from build123d import *

# Parameters (mm, degrees)
SKETCH1_W                 = 146.05
SKETCH1_H                 = 266.7
BOSS_EXTRUDE1_DEPTH       = 15.875
SKETCH2_W                 = 110.49
SKETCH2_H                 = 224.79
CUT_EXTRUDE1_DEPTH        = 2.54
CUT_EXTRUDE2_DEPTH        = 10.16
F_4_40_TAPPED_HOLE1_D     = 2.2606
F_4_40_TAPPED_HOLE1_DEPTH = 10.16
F_4_40_TAPPED_HOLE1_TIP   = 0.679152758
F_8_CLEARANCE_HOLE1_D     = 4.9149
F_8_32_TAPPED_HOLE1_D     = 3.4544
F_8_32_TAPPED_HOLE1_DEPTH = 12.7
F_8_32_TAPPED_HOLE1_TIP   = 1.037806461
F_4_40_TAPPED_HOLE2_D     = 2.2606
F_4_40_TAPPED_HOLE2_DEPTH = 10.16
F_4_40_TAPPED_HOLE2_TIP   = 0.679152758


with BuildPart() as part:
    # Sketch1 → Boss-Extrude1 (new body)
    with BuildSketch(Plane(origin=(0, 0, 0), x_dir=(1, 0, 0), z_dir=(0, 1, 0))):
        with Locations((73.025, 133.35)):
            Rectangle(SKETCH1_W, SKETCH1_H)
    extrude(amount=BOSS_EXTRUDE1_DEPTH)

    # Sketch2 → Cut-Extrude1 (cut)
    with BuildSketch(Plane(origin=(0, 15.875, 0), x_dir=(1, 0, 0), z_dir=(0, 1, 0))):
        with Locations((60.96, 130.81)):
            Rectangle(SKETCH2_W, SKETCH2_H)
    extrude(amount=-CUT_EXTRUDE1_DEPTH, mode=Mode.SUBTRACT)

    # Sketch3 → Cut-Extrude2 (cut)
    with BuildSketch(Plane(origin=(0, 13.335, 0), x_dir=(1, 0, 0), z_dir=(0, 1, 0))):
        Polygon((19.685, 26.035), (19.685, 18.415), (5.715, 18.415), (5.715, 32.385), (13.335, 32.385), (13.335, 121.285), (19.685, 121.285), (19.685, 133.985), (5.715, 133.985), (5.715, 243.205), (19.685, 243.205), (19.685, 235.585), (37.8587, 235.585), (37.8587, 26.035), align=None)
        Polygon((44.2087, 26.035), (102.235, 26.035), (102.235, 18.415), (116.205, 18.415), (116.205, 32.385), (108.585, 32.385), (108.585, 121.285), (102.235, 121.285), (102.235, 133.985), (108.585, 133.985), (108.585, 229.235), (116.205, 229.235), (116.205, 243.205), (102.235, 243.205), (102.235, 235.585), (44.2087, 235.585), align=None)
    extrude(amount=-CUT_EXTRUDE2_DEPTH, mode=Mode.SUBTRACT)

    # #4-40 Tapped Hole1
    with Locations(Plane(origin=(0, 13.335, 0), x_dir=(1, 0, 0), z_dir=(0, 1, 0))):
        with Locations((108.585, 127.635), (13.335, 127.635)):
            Hole(F_4_40_TAPPED_HOLE1_D / 2, depth=F_4_40_TAPPED_HOLE1_DEPTH)
            with Locations((0, 0, -(F_4_40_TAPPED_HOLE1_DEPTH + F_4_40_TAPPED_HOLE1_TIP / 2))):  # 118° drill point
                Cone(0, F_4_40_TAPPED_HOLE1_D / 2, F_4_40_TAPPED_HOLE1_TIP, mode=Mode.SUBTRACT)

    # #8 Clearance Hole1 (through all)
    with Locations(Plane(origin=(0, 15.875, 0), x_dir=(1, 0, 0), z_dir=(0, 1, 0))):
        with Locations((12.7, 6.35), (139.7, 6.35), (139.7, 260.35), (12.7, 260.35)):
            Hole(F_8_CLEARANCE_HOLE1_D / 2)

    # #8-32 Tapped Hole1
    with Locations(Plane(origin=(0, 15.875, 0), x_dir=(1, 0, 0), z_dir=(0, 1, 0))):
        with Locations((44.2087, 6.35), (44.2087, 260.35), (139.7, 133.35)):
            Hole(F_8_32_TAPPED_HOLE1_D / 2, depth=F_8_32_TAPPED_HOLE1_DEPTH)
            with Locations((0, 0, -(F_8_32_TAPPED_HOLE1_DEPTH + F_8_32_TAPPED_HOLE1_TIP / 2))):  # 118° drill point
                Cone(0, F_8_32_TAPPED_HOLE1_D / 2, F_8_32_TAPPED_HOLE1_TIP, mode=Mode.SUBTRACT)

    # #4-40 Tapped Hole2
    with Locations(Plane(origin=(0, 15.875, 0), x_dir=(1, 0, 0), z_dir=(0, 1, 0))):
        with Locations((108.585, 249.555), (122.555, 26.035), (25.4, 249.555), (25.4, 12.065)):
            Hole(F_4_40_TAPPED_HOLE2_D / 2, depth=F_4_40_TAPPED_HOLE2_DEPTH)
            with Locations((0, 0, -(F_4_40_TAPPED_HOLE2_DEPTH + F_4_40_TAPPED_HOLE2_TIP / 2))):  # 118° drill point
                Cone(0, F_4_40_TAPPED_HOLE2_D / 2, F_4_40_TAPPED_HOLE2_TIP, mode=Mode.SUBTRACT)


solid = part.part
Geometry check sheet. Reference: the model listing, model coordinates, mm. A direction names the side the tool comes from. Give positions to 0.01 mm unless a question says otherwise; leave off trailing zeros. Order: outer loops, then holes, each group sorted by start corner. A loop starts at its lowest first (then second) coordinate and runs counter-clockwise, first axis right, second up. Notation, with made-up numbers: M 72,26 L 91,26 A34 ccw 91,61 Z; hole C 11.5,44 d11. An arc over 180 degrees is marked long. Use a Markdown table: item, result.
Item 1: Draft check along X on faces 3 (the flat face through (121, 15.875, -135)), 4 (the cylindrical face through (14.51, 7.83, -8.01)). Enter one of: +X half, -X half, draft (parallel to the pull), parting line (faces both ways), or undercut.
Answers follow:
| item | result |
|---|---|
| face 3 | draft |
| face 4 | undercut |
Item 2: Material ranges on line 1 along X through (y, z) = (7.75, -197.5) (3 decimals); line 2 along Z through (x, y) = (14.5, 14) (3 decimals); line 3 along Z through (x, y) = (11, 10.5) (3 decimals), recorded low to high.
Answers follow:
| item | result |
|---|---|
| line 1 | x = 0 to 5.715, 37.859 to 44.209, 108.585 to 146.05 |
| line 2 | z = -266.7 to -262.023, -258.677 to -243.205, -18.415 to -8.023, -4.677 to 0 |
| line 3 | z = -266.7 to -262.125, -258.575 to -243.205, -133.985 to -32.385, -18.415 to -8.125, -4.575 to 0 |
Item 3: Section check B-B (z = -222.5). Record the cut outline in (x, y) (3 decimals).
Answers follow:
| item | result |
|---|---|
| outline | M 0,0 L 146.05,0 L 146.05,15.875 L 116.205,15.875 L 116.205,13.335 L 108.585,13.335 L 108.585,3.175 L 44.209,3.175 L 44.209,13.335 L 37.859,13.335 L 37.859,3.175 L 5.715,3.175 L 5.715,15.875 L 0,15.875 Z |
Item 4: Depth check by flat-ended pin: P1, Ø6, axis at x = 43.5, z = -161.5, coming from the +Y side (3 decimals); P2, Ø2, axis at x = 34.5, z = -216.5, coming from the +Y side (3 decimals); P3, Ø4, axis at x = 12.7, z = -6.35, coming from the +Y side. Enter the tip coordinate at first touch or a pass-through.
Answers follow:
| item | result |
|---|---|
| P1 | stops at y = 13.335 |
| P2 | stops at y = 3.175 |
| P3 | passes through |
Item 5: Section check C-C (z = -58.5). Record the cut outline in (x, y) (3 decimals).
Answers follow:
| item | result |
|---|---|
| outline | M 0,0 L 146.05,0 L 146.05,15.875 L 116.205,15.875 L 116.205,13.335 L 108.585,13.335 L 108.585,3.175 L 44.209,3.175 L 44.209,13.335 L 37.859,13.335 L 37.859,3.175 L 13.335,3.175 L 13.335,13.335 L 5.715,13.335 L 5.715,15.875 L 0,15.875 Z |
Item 6: Tool access check on faces 1 (the flat face through (73, 8, -26.035)), 2 (the flat face through (72, 8, -266.7)). Record the directions out of +Z, -Z, +X, -X, +Y, -Y that give a thin tool (end or side, any length) a straight path to the whole face; none if there is none.
Answers follow:
| item | result |
|---|---|
| face 1 | +Y |
| face 2 | -Z, +X, -X, +Y, -Y |
Item 7: Section check D-D (y = 10.25). State how many separate pieces and enclosed holes the cut face has, and give its area (3 significant figures).
Answers follow:
| item | result |
|---|---|
| separate pieces | 1 |
| enclosed holes | 15 |
| area | 19,000 mm2 |
Item 8: Section check A-A (x = 87.5). Record the cut outline in (y, z) (3 decimals).
Answers follow:
| item | result |
|---|---|
| outline | M 0,-266.7 L 15.875,-266.7 L 15.875,-243.205 L 13.335,-243.205 L 13.335,-235.585 L 3.175,-235.585 L 3.175,-26.035 L 13.335,-26.035 L 13.335,-18.415 L 15.875,-18.415 L 15.875,0 L 0,0 Z |
